Design review of the part shown in the three views and the two pictorial views. Dimensions are in mm from the part's minimum x, y and z. Give positions to 0.01 mm unless a question says otherwise; leave off trailing zeros. Loops run counter-clockwise (first coordinate to the right, second up) from the corner with the lowest first, then second, coordinate; pieces in that order, holes last. Notation, with made-up numbers: (19.5, -30.5) -> (31.5, -30.5) arc R29 cw to (31.5, -6.5) -> close; hole circle Ø7 at (79.5, -3.75). An arc over 180 degrees is marked (long way). Use CSV: the item, a comma, the result in double quotes. Start each with the question number.
Item 1: We need section C-C (x = 13.5). State the section outline as (y, z) points (1 decimal).
Item 2: Wall thickness on line 1 along Y through (x, z) = (2.5, 63); line 2 along X through (y, z) = (47, 86.5) (1 decimal); line 3 along Z through (x, y) = (11, 23.5) (1 decimal): over which ranges is each line inside the solid? List them lowest first. Write a range as from..to.
Item 3: Clearance check with flat-ended pins moving along their axes: pin 1 (5.5 mm diameter, centred on x = 11.11, y = 19.05, fed in from +Z) (1 decimal); pin 2 (11.5 mm diameter, centred on y = 56, z = 69.5, fed in from -X). State where each tip first meets the part, or that it passes through.
Item 4: We need section D-D (y = 51.5). State the section outline as (x, z) points (1 decimal), plus the area to 3 significant figures.
Item 5: We need section B-B (z = 57). State the section outline as (x, y) points (1 decimal).
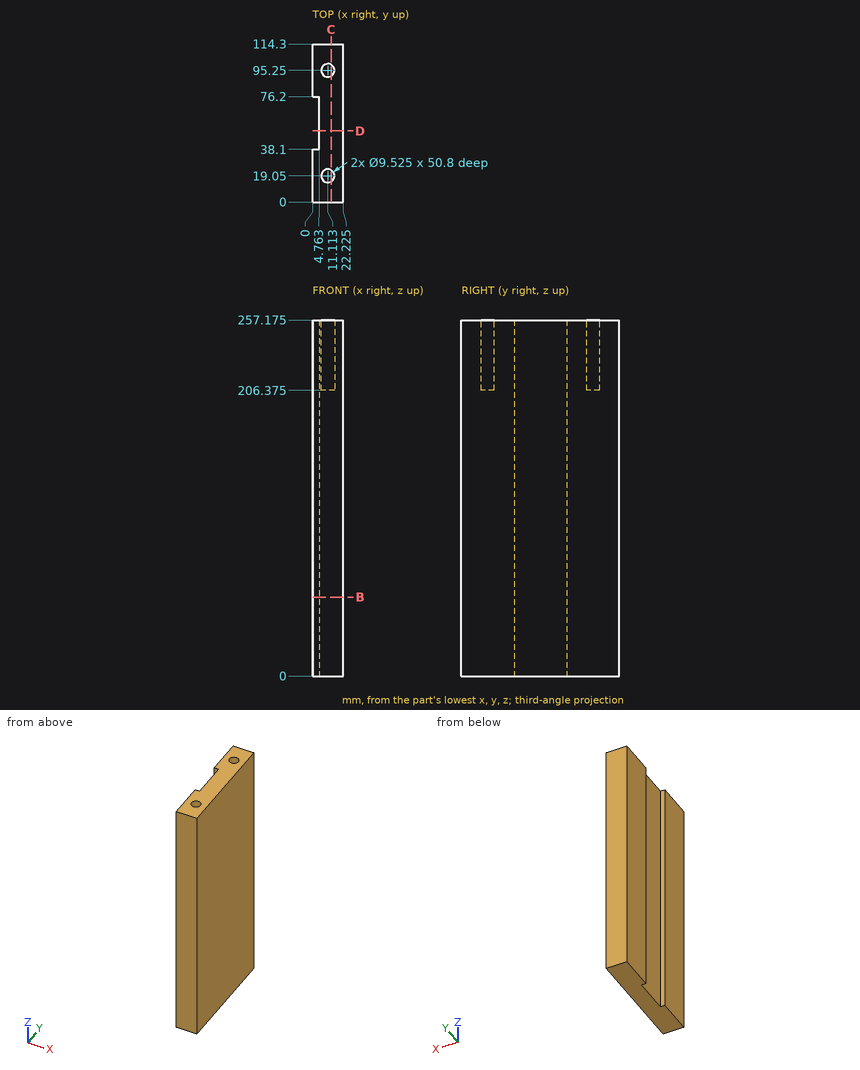
Results found:
1,outline,"(0, 0) -> (114.3, 0) -> (114.3, 257.2) -> (99.4, 257.2) -> (99.4, 206.4) -> (91.1, 206.4) -> (91.1, 257.2) -> (23.2, 257.2) -> (23.2, 206.4) -> (14.9, 206.4) -> (14.9, 257.2) -> (0, 257.2) -> close"
2,line 1,"0..38.1, 76.2..114.3"
2,line 2,"4.8..22.2"
2,line 3,"0..206.4"
3,pin 1,"z = 206.4"
3,pin 2,"x = 4.76"
4,outline,"(4.8, 0) -> (22.2, 0) -> (22.2, 257.2) -> (4.8, 257.2) -> close"
4,area,"4,490 mm²"
5,outline,"(0, 0) -> (22.2, 0) -> (22.2, 114.3) -> (0, 114.3) -> (0, 76.2) -> (4.8, 76.2) -> (4.8, 38.1) -> (0, 38.1) -> close"
